Here's how the part is built. I have some questions about the finished solid (model axes, mm). A direction names the side the tool comes from. Round coordinates to 2 decimals unless told otherwise and drop trailing zeros. Write each loop counter-clockwise with the first axis right and the second up, starting at its lowest first coordinate (ties: lowest second). Pieces come first, ordered by that corner, then holes. Notation, with made-up numbers: M 71,53 L 125,53 A18 cw 125,62 Z; hole C -37.75,-10.5 d2. An arc over 180 degrees is marked long. Write item = value, one per line. Start each with the question number.
(1) Will these pins go through, and if not, where does the flat tip stop? pin 1 Ø0.8 at (y, z) = (3, -5.5) entering from -X; pin 2 Ø1.8 at (x, y) = (-1.02, -0.72) entering from -Z; pin 3 Ø0.5 at (x, z) = (0.5, -4) entering from -Y.
(2) If we mould it in two halves opening along X, with no side actions, what happens to faces 5 (the flat face through (-28, 3, -5.97)), 6 (the flat face through (-30.557, 3, -5)), 7 (the cylindrical face through (-0.066, -0.42, -4.064))? For each: released by +X, released by -X, zero draft, split by the parting line, or undercut.
(3) I want a section at A-A (y = 3.1). List the corners of the cut face in (x, z) for me, and give its area (3 significant figures).
(4) On a 3-axis mill with a long thin cutter (end or side, diameter ignored), from which of +Z, -Z, +X, -X, +Y, -Y can I reach the whole of each face in a straight line? I mean faces 1 (the flat face through (-21, 1.028, -5)), 2 (the flat face through (-28, 1.367, -5)), 3 (the flat face through (-19.856, 3, -5)), 4 (the flat face through (-21, 4.079, -5)). Say none if no direction works.
(5) I need wall thicknesses on line 1 along Y through (x, z) = (-26.19, -4.15); line 2 along Y through (x, z) = (-1.02, -4); line 3 along X through (y, z) = (1.75, -5.2). Which ranges of each line are inside material? Lowest first, please.
(6) I want a section at B-B (x = -37.5). List the corners of the cut face in (y, z) for me.
```python
from build123d import *

# Parameters (mm, degrees)
BOSS_EXTRUDE1_DEPTH = 0.8
SKETCH2_W           = 2.797017598
SKETCH2_H           = 3.051291925
SKETCH2_W_2         = 4.216715925
SKETCH2_H_2         = 2.39441658
BOSS_EXTRUDE2_DEPTH = 1.5


with BuildPart() as part:
    # Sketch1 → Boss-Extrude1 (new body)
    with BuildSketch(Plane.XY.offset(-3.67)):
        with BuildLine():
            Line((-47.1, 0.52), (-46.5, 0.52))
            ThreePointArc((-46.5, 0.52), (-45.95, -0.03), (-46.5, -0.58))
            Line((-46.5, -0.58), (-47.1, -0.58))
            ThreePointArc((-47.1, -0.58), (-47.241421356, -0.638578644), (-47.3, -0.78))
            Line((-47.3, -0.78), (-47.3, -1.9))
            ThreePointArc((-47.3, -1.9), (-47.153553391, -2.253553391), (-46.8, -2.4))
            Line((-46.8, -2.4), (0.2, -2.4))
            ThreePointArc((0.2, -2.4), (0.553553391, -2.253553391), (0.7, -1.9))
            Line((0.7, -1.9), (0.7, 2.35))
            ThreePointArc((0.7, 2.35), (0.641421356, 2.491421356), (0.5, 2.55))
            Line((0.5, 2.55), (-0.1, 2.55))
            ThreePointArc((-0.1, 2.55), (-0.65, 3.1), (-0.1, 3.65))
            Line((-0.1, 3.65), (0.5, 3.65))
            ThreePointArc((0.5, 3.65), (0.641421356, 3.708578644), (0.7, 3.85))
            Line((0.7, 3.85), (0.7, 8.1))
            ThreePointArc((0.7, 8.1), (0.553553391, 8.453553391), (0.2, 8.6))
            Line((0.2, 8.6), (-46.8, 8.6))
            ThreePointArc((-46.8, 8.6), (-47.153553391, 8.453553391), (-47.3, 8.1))
            Line((-47.3, 8.1), (-47.3, 0.72))
            ThreePointArc((-47.3, 0.72), (-47.241421356, 0.578578644), (-47.1, 0.52))
        make_face()
        with BuildLine():
            ThreePointArc((-2.02, -0.72), (-1.02, -1.72), (-0.02, -0.72))
            ThreePointArc((-0.02, -0.72), (-1.02, 0.28), (-2.02, -0.72))
        make_face(mode=Mode.SUBTRACT)
        with BuildLine():
            ThreePointArc((-27.19, 0.1), (-26.19, -0.9), (-25.19, 0.1))
            ThreePointArc((-25.19, 0.1), (-26.19, 1.1), (-27.19, 0.1))
        make_face(mode=Mode.SUBTRACT)
    extrude(amount=-BOSS_EXTRUDE1_DEPTH)

    # Sketch2 → Boss-Extrude2 (add)
    with BuildSketch(Plane(origin=(0, 0, -4.47), x_dir=(-1, 0, 0), z_dir=(0, 0, -1))):
        with Locations((21.254561383, 2.553733594)):
            Rectangle(SKETCH2_W, SKETCH2_H)
        with Locations((28.448405888, 2.564328357)):
            Rectangle(SKETCH2_W_2, SKETCH2_H_2)
    extrude(amount=BOSS_EXTRUDE2_DEPTH)


solid = part.part
```
Returned:
q1.pin_1 = -30.56
q1.pin_2 = through
q1.pin_3 = -2.4
q2.face_5 = zero draft
q2.face_6 = released by -X
q2.face_7 = undercut
q3.outline = M -47.3,-4.47 L -30.56,-4.47 L -30.56,-5.97 L -26.34,-5.97 L -26.34,-4.47 L -22.65,-4.47 L -22.65,-5.97 L -19.86,-5.97 L -19.86,-4.47 L -0.65,-4.47 L -0.65,-3.67 L -47.3,-3.67 Z
q3.area = 47.8 mm²
q4.face_1 = -Z, +X, -X, -Y
q4.face_2 = -Z, -X, -Y
q4.face_3 = -Z, +X, +Y, -Y
q4.face_4 = -Z, +X, -X, +Y
q5.line_1 = -2.4 to -0.9, 1.1 to 8.6
q5.line_2 = -2.4 to -1.72, 0.28 to 8.6
q5.line_3 = -30.56 to -26.34, -22.65 to -19.86
q6.outline = M -2.4,-4.47 L 8.6,-4.47 L 8.6,-3.67 L -2.4,-3.67 Z
